from build123d import *

# Parameters (mm, degrees)
RESSALTO_EXTRUS_O1_DEPTH = 30
FILETE1_R                = 0.2
ESBO_O2_R                = 1.0922
RESSALTO_EXTRUS_O2_DEPTH = 6
ESBO_O3_R                = 1.0922
CORTE_EXTRUS_O1_DEPTH    = 4.76


with BuildPart() as part:
    # Esboço1 → Ressalto-extrusão1 (new body)
    with BuildSketch(Plane(origin=(0, 0, 0), x_dir=(1, 0, 0), z_dir=(0, 1, 0))):
        Polygon((2.886751346, 0), (1.443375673, 2.5), (-1.443375673, 2.5), (-2.886751346, 0), (-1.443375673, -2.5), (1.443375673, -2.5), align=None)
    extrude(amount=RESSALTO_EXTRUS_O1_DEPTH)

    # Filete1
    filete1_edges = [part.edges().sort_by_distance(p)[0] for p in [
        (0, 30, -2.5),
        (-2.165063509, 30, -1.25),
        (-2.165063509, 30, 1.25),
        (0, 30, 2.5),
        (2.165063509, 30, 1.25),
        (0, 0, 2.5),
        (-2.165063509, 0, 1.25),
        (-2.165063509, 0, -1.25),
        (2.165063509, 30, -1.25),
        (0, 0, -2.5),
        (2.165063509, 0, -1.25),
        (2.165063509, 0, 1.25),
    ]]
    fillet(filete1_edges, radius=FILETE1_R)

    # Esboço2 → Ressalto-extrusão2 (add)
    with BuildSketch(Plane.XZ):
        with Locations(Location((0, 0, 0), (0, 0, 90))):
            Circle(ESBO_O2_R)
    extrude(amount=RESSALTO_EXTRUS_O2_DEPTH)

    # Esboço3 → Corte-extrusão1 (cut)
    with BuildSketch(Plane(origin=(0, 30, 0), x_dir=(1, 0, 0), z_dir=(0, 1, 0))):
        with Locations(Location((0, 0, 0), (0, 0, 270))):
            Circle(ESBO_O3_R)
    extrude(amount=-CORTE_EXTRUS_O1_DEPTH, mode=Mode.SUBTRACT)


solid = part.part
Here's how the part is built. I have some questions about the finished solid (model axes, mm). A direction names the side the tool comes from. Coordinates: 2 decimals unless noted, no trailing zeros. Write each loop counter-clockwise with the first axis right and the second up, starting at its lowest first coordinate (ties: lowest second). Pieces come first, ordered by that corner, then holes.
Item 1: On a 3-axis mill with a long thin cutter (end or side, diameter ignored), from which of +Z, -Z, +X, -X, +Y, -Y can I reach the whole of each face in a straight line? I mean faces 1 (the cylindrical face through (0.33, 27.65, 1.04)), 2 (the flat face through (1, 0, -1)), 3 (the cylindrical face through (-2.106, 29.94, 1.239)). Say none if no direction works.
Item 2: I want a section at A-A on y = 26. Write out the boundary of the cut face in (x, z).
Item 3: Will this pin go through, and if not, where does the flat tip stop? pin 1 (0.7 mm diameter, centred on x = -0.5, z = 0, fed in from +Y).
Item 4: I want a section at C-C on y = -1. Write out the boundary of the cut face in (x, z), and give its area (3 significant figures).
Item 5: I want a section at B-B on x = 0. Write out the boundary of the cut face in (y, z), and give its area (3 significant figures).
Item 6: If I drill on line 1 (Y direction, x = 0.7, z = -1); line 2 (Y direction, x = 0.15, z = -0.3); line 3 (Z direction, x = 2.05, y = 7), over which ranges is the centre line in solid material (lowest first)?
Item 7: If we mould it in two halves opening along X, with no side actions, what happens to faces 4 (the flat face through (0, 25.24, 0)), 5 (the cylindrical face through (-0.33, -2.96, 1.04)), 6 (the cylindrical face through (2.13, 0.06, 1.2)), 7 (the flat face through (0, 15, -2.5))? For each: +X half, -X half, draft (parallel to the pull), parting line (faces both ways), or undercut.
Findings below:
1. face 1: +Y
1. face 2: -Y
1. face 3: +Z, -X, +Y
2. outline: (-2.89, 0) - (-1.44, -2.5) - (1.44, -2.5) - (2.89, 0) - (1.44, 2.5) - (-1.44, 2.5) - close; hole circle Ø2.18 at (0, 0)
3. pin 1: stops at y = 25.24
4. outline: circle Ø2.18 at (0, 0)
4. area: 3.75 mm2
5. outline: (-6, -1.09) - (0, -1.09) - (0, -2.3) arc R0.2 ccw to (0.2, -2.5) - (29.8, -2.5) arc R0.2 ccw to (30, -2.3) - (30, -1.09) - (25.24, -1.09) - (25.24, 1.09) - (30, 1.09) - (30, 2.3) arc R0.2 ccw to (29.8, 2.5) - (0.2, 2.5) arc R0.2 ccw to (0, 2.3) - (0, 1.09) - (-6, 1.09) - close
5. area: 153 mm2
6. line 1: y = 0 to 30
6. line 2: y = -6 to 25.24
6. line 3: z = -1.45 to 1.45
7. face 4: undercut
7. face 5: parting line
7. face 6: +X half
7. face 7: draft
